Here's how the part is built. I have some questions about the finished solid (model axes, mm). Face numbers are marked on the shaded views. A direction names the side the tool comes from. Round coordinates to 2 decimals unless told otherwise and drop trailing zeros. Write each loop counter-clockwise with the first axis right and the second up, starting at its lowest first coordinate (ties: lowest second). Pieces come first, ordered by that corner, then holes. Notation, with made-up numbers: (8.25, 82) - (28.25, 82) arc R21 cw to (28.25, 106) - close; hole circle Ø3 at (8, 55.5). An arc over 180 degrees is marked (long way). One line per item, written item: value. Start each with the question number.
Item 1: For the marked faces 1, 2, 3, 4 and 5, which set-ups out of +Z, -Z, +X, -X, +Y, -Y let a thin tool reach every point of the face, with its end or its side?
Item 2: If I drill on line 1 (X direction, y = 32, z = 17); line 2 (X direction, y = 52, z = 28.5) (3 decimals); line 3 (Z direction, x = 31.5, y = 6.5), over which ranges is the centre line in solid material (lowest first)?
Item 3: Imagine slicing it at B-B, the plane z = 40. Please give me the cut outline in (x, y) (3 decimals), then the cut area to 3 significant figures.
Item 4: Thinking about a two-plate mould opening in Y: for the marked faces 6, 7, 8 and 9, which applies, released by +Y, released by -Y, zero draft, split by the parting line, or undercut?
Item 5: Imagine slicing it at C-C, the plane y = 26. Please give me the cut outline in (x, z) (1 decimal), then the cut area to 3 significant figures.
Item 6: Imagine slicing it at A-A, the plane z = 28. Please give me the cut outline in (x, y) (3 decimals), then the cut area to 3 significant figures.
Item 7: For P1, Ø6, axis at x = 77, y = 13.5, coming from the +Z side; P2, Ø5, axis at x = 9, y = 21.5, coming from the +Z side; P3, Ø9, axis at y = 24.5, z = 30, coming from the +X side (3 decimals), each with a flat end and sliding along its axis, tell me the tip position at first contact or that it passes through.
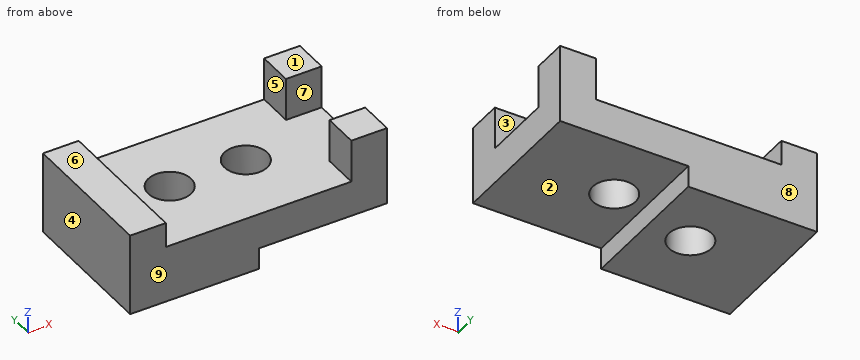
```python
from build123d import *

# Parameters (mm, degrees)
F0_W      = 114.3
F0_H      = 63.5
F1_DEPTH  = 36.5125
F2_W      = 114.3
F2_H      = 63.5
F3_DEPTH  = 11.1125
F4_W      = 57.1499951184
F4_H      = 64.068160916
F5_DEPTH  = 9.525
F6_W      = 15.875
F6_H      = 15.875
F7_DEPTH  = 19.05
F8_W      = 15.875
F8_H      = 15.875
F9_DEPTH  = 19.05
F10_W     = 15.875
F10_H     = 63.5
F11_DEPTH = 11.1125
F12_R     = 9.525
F13_DEPTH = 25.4
F14_R     = 9.525
F15_DEPTH = 25.4


with BuildPart() as f1:
    # F0 (on Top) → F1 (new body)
    with BuildSketch(Plane.XY):
        with Locations((57.15, 31.75)):
            Rectangle(F0_W, F0_H)
    extrude(amount=F1_DEPTH)

    # F2 (on face) → F3 (cut)
    with BuildSketch(Plane.XY.offset(36.5125)):
        with Locations((57.15, 31.75)):
            Rectangle(F2_W, F2_H)
    extrude(amount=-F3_DEPTH, mode=Mode.SUBTRACT)

    # F4 (on Top) → F5 (cut)
    with BuildSketch(Plane.XY):
        with Locations((85.8252625912, 32.034080458)):
            Rectangle(F4_W, F4_H)
    extrude(amount=F5_DEPTH, mode=Mode.SUBTRACT)

    # F6 (on face) → F7 (join)
    with BuildSketch(Plane.XY.offset(25.4)):
        with Locations((106.3625, 7.9375)):
            Rectangle(F6_W, F6_H)
    extrude(amount=F7_DEPTH)

    # F8 (on face) → F9 (join)
    with BuildSketch(Plane.XY.offset(25.4)):
        with Locations((106.3625, 55.5625)):
            Rectangle(F8_W, F8_H)
    extrude(amount=F9_DEPTH)

    # F10 (on face) → F11 (join)
    with BuildSketch(Plane.XY.offset(25.4)):
        with Locations((7.9375, 31.75)):
            Rectangle(F10_W, F10_H)
    extrude(amount=F11_DEPTH)

    # F12 (on face) → F13 (cut)
    with BuildSketch(Plane.XY.offset(25.4)):
        with Locations((37.9997342825, 33.3876311779)):
            Circle(F12_R)
    extrude(amount=-F13_DEPTH, mode=Mode.SUBTRACT)

    # F14 (on face) → F15 (cut)
    with BuildSketch(Plane.XY.offset(25.4)):
        with Locations((71.6881528497, 33.0868437886)):
            Circle(F14_R)
    extrude(amount=-F15_DEPTH, mode=Mode.SUBTRACT)


solid = f1.part
```
Values follow:
1. face 1: +Z, +X, -X, +Y, -Y
1. face 2: -Z, +X, +Y, -Y
1. face 3: +Z, +X
1. face 4: +Z, -Z, -X, +Y, -Y
1. face 5: +Z, +Y, -Y
2. line 1: x = 0 to 28.58, 47.42 to 62.23, 81.15 to 114.3
2. line 2: x = 0 to 15.875, 98.425 to 114.3
2. line 3: z = 0 to 25.4
3. outline: (98.425, 0) - (114.3, 0) - (114.3, 15.875) - (98.425, 15.875) - close; (98.425, 47.625) - (114.3, 47.625) - (114.3, 63.5) - (98.425, 63.5) - close
3. area: 504 mm^2
4. face 6: zero draft
4. face 7: undercut
4. face 8: released by +Y
4. face 9: released by -Y
5. outline: (0, 0) - (32, 0) - (32, 25.4) - (15.9, 25.4) - (15.9, 36.5) - (0, 36.5) - close; (44, 0) - (57.3, 0) - (57.3, 9.5) - (65.3, 9.5) - (65.3, 25.4) - (44, 25.4) - close; (78.1, 9.5) - (114.3, 9.5) - (114.3, 25.4) - (78.1, 25.4) - close
5. area: 2,030 mm^2
6. outline: (0, 0) - (15.875, 0) - (15.875, 63.5) - (0, 63.5) - close; (98.425, 0) - (114.3, 0) - (114.3, 15.875) - (98.425, 15.875) - close; (98.425, 47.625) - (114.3, 47.625) - (114.3, 63.5) - (98.425, 63.5) - close
6. area: 1,510 mm^2
7. P1: stops at z = 25.4
7. P2: stops at z = 36.51
7. P3: stops at x = 15.875
